from build123d import *

# Parameters (mm, degrees)
ESQUISSE1_W             = 15.74
ESQUISSE1_H             = 2.54
BOSS_EXTRU_1_DEPTH      = 8.5
ESQUISSE3_W             = 0.626711562
ESQUISSE3_H             = 0.626711562
ENL_V_MAT_EXTRU_3_DEPTH = 8
CHANFREIN3_SIZE         = 0.6
CHANFREIN3_SIZE2        = 0.267137211
ESQUISSE6_W             = 0.75
ESQUISSE6_H             = 0.4
BOSS_EXTRU_3_DEPTH      = 3.2
CONG_1_R                = 0.3


with BuildPart() as part:
    # Esquisse1 → Boss.-Extru.1 (new body)
    with BuildSketch(Plane(origin=(0, 0, 0), x_dir=(1, 0, 0), z_dir=(0, 1, 0))):
        Rectangle(ESQUISSE1_W, ESQUISSE1_H)
    extrude(amount=BOSS_EXTRU_1_DEPTH)

    # Esquisse3 → Enlèv. mat.-Extru.3 (cut)
    with BuildSketch(Plane(origin=(0, 8.5, 0), x_dir=(1, 0, 0), z_dir=(0, 1, 0))):
        with Locations((-6.35, 0)):
            Rectangle(ESQUISSE3_W, ESQUISSE3_H)
        with Locations((-3.81, 0)):
            Rectangle(ESQUISSE3_W, ESQUISSE3_H)
        with Locations((-1.27, 0)):
            Rectangle(ESQUISSE3_W, ESQUISSE3_H)
        with Locations((1.27, 0)):
            Rectangle(ESQUISSE3_W, ESQUISSE3_H)
        with Locations((3.81, 0)):
            Rectangle(ESQUISSE3_W, ESQUISSE3_H)
        with Locations((6.35, 0)):
            Rectangle(ESQUISSE3_W, ESQUISSE3_H)
    extrude(amount=-ENL_V_MAT_EXTRU_3_DEPTH, mode=Mode.SUBTRACT)

    # Chanfrein3
    chanfrein3_edges = [part.edges().sort_by_distance(p)[0] for p in [
        (-3.81, 8.5, -0.313355781),
        (-3.496644219, 8.5, 0),
        (-4.123355781, 8.5, 0),
        (-3.81, 8.5, 0.313355781),
        (-6.35, 8.5, -0.313355781),
        (-6.036644219, 8.5, 0),
        (-6.663355781, 8.5, 0),
        (-6.35, 8.5, 0.313355781),
        (3.81, 8.5, -0.313355781),
        (4.123355781, 8.5, 0),
        (3.496644219, 8.5, 0),
        (3.81, 8.5, 0.313355781),
        (1.27, 8.5, -0.313355781),
        (1.583355781, 8.5, 0),
        (0.956644219, 8.5, 0),
        (1.27, 8.5, 0.313355781),
        (-1.27, 8.5, -0.313355781),
        (-0.956644219, 8.5, 0),
        (-1.583355781, 8.5, 0),
        (-1.27, 8.5, 0.313355781),
        (6.35, 8.5, -0.313355781),
        (6.663355781, 8.5, 0),
        (6.036644219, 8.5, 0),
        (6.35, 8.5, 0.313355781),
    ]]
    chanfrein3_side = [part.faces().sort_by_distance(p)[0] for p in [
        (0, 8.5, 0),
    ]]
    chamfer(chanfrein3_edges, length=CHANFREIN3_SIZE, length2=CHANFREIN3_SIZE2, reference=chanfrein3_side[0])

    # Esquisse6 → Boss.-Extru.3 (add)
    with BuildSketch(Plane.XZ):
        with Locations((-6.35, 0)):
            Rectangle(ESQUISSE6_W, ESQUISSE6_H)
        with Locations((-3.81, 0)):
            Rectangle(ESQUISSE6_W, ESQUISSE6_H)
        with Locations((-1.27, 0)):
            Rectangle(ESQUISSE6_W, ESQUISSE6_H)
        with Locations((1.27, 0)):
            Rectangle(ESQUISSE6_W, ESQUISSE6_H)
        with Locations((3.81, 0)):
            Rectangle(ESQUISSE6_W, ESQUISSE6_H)
        with Locations((6.35, 0)):
            Rectangle(ESQUISSE6_W, ESQUISSE6_H)
    extrude(amount=BOSS_EXTRU_3_DEPTH)

    # Congé1
    cong_1_edges = [part.edges().sort_by_distance(p)[0] for p in [
        (-5.975, -3.2, 0),
        (-6.725, -3.2, 0),
        (-3.435, -3.2, 0),
        (-4.185, -3.2, 0),
        (-0.895, -3.2, 0),
        (-1.645, -3.2, 0),
        (1.645, -3.2, 0),
        (0.895, -3.2, 0),
        (4.185, -3.2, 0),
        (3.435, -3.2, 0),
        (6.725, -3.2, 0),
        (5.975, -3.2, 0),
    ]]
    fillet(cong_1_edges, radius=CONG_1_R)


solid = part.part
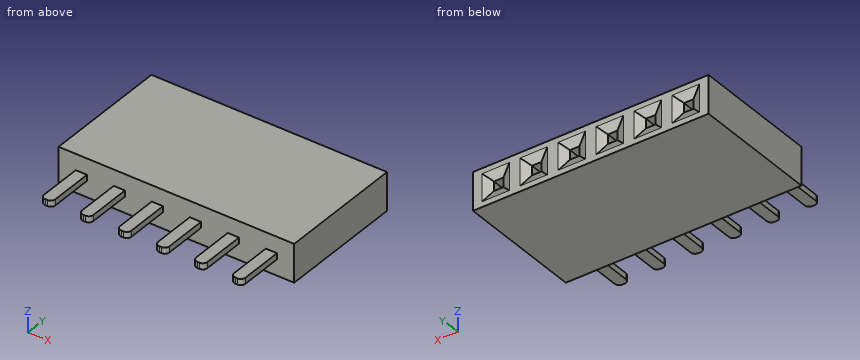
Verification items for the finished model (mm, model axes). Coordinates: 2 decimals unless noted, no trailing zeros. Order: outer loops, then holes, each group sorted by start corner. A loop starts at its lowest first (then second) coordinate and runs counter-clockwise, first axis right, second up. Notation, with made-up numbers: M 13,65.25 L 59,65.25 A31 ccw 59,91.25 Z; hole C 31.25,67 d11. An arc over 180 degrees is marked long. One line per item, written item: value. Start each with the question number.
Item 1: Scan lines: probe 1 along Z at (x, y) = (1.5, 6); probe 2 along Y at (x, z) = (5.75, -1.2); probe 3 along Y at (x, z) = (1.25, 0). Record each from-to range of solid material in increasing order.
Item 2: Sectioned sample at B-B (y = -1.5). Enter the section's corners in (x, z) (3 decimals).
Item 3: Gauge pin test, flat ends, axial feed: pin 1 (0.8 mm diameter, centred on x = 1, y = -1.5, fed in from -Z); pin 2 (0.6 mm diameter, centred on x = 6.5, y = -2, fed in from +Z). Record the tip position at first contact, or that the pin passes through.
Item 4: Sectioned sample at C-C (z = 0.65). Enter the section's corners in (x, y), then the cut area to 3 significant figures.
Item 5: Sectioned sample at A-A (y = 2). Enter the section's corners in (x, z), then the cut area to 3 significant figures.
Conclusion:
1. probe 1: z = -1.27 to -0.31, 0.31 to 1.27
1. probe 2: y = 0 to 8.5
1. probe 3: y = -3.2 to 0.5
2. outline: M -6.725,-0.2 L -5.975,-0.2 L -5.975,0.2 L -6.725,0.2 Z; M -4.185,-0.2 L -3.435,-0.2 L -3.435,0.2 L -4.185,0.2 Z; M -1.645,-0.2 L -0.895,-0.2 L -0.895,0.2 L -1.645,0.2 Z; M 0.895,-0.2 L 1.645,-0.2 L 1.645,0.2 L 0.895,0.2 Z; M 3.435,-0.2 L 4.185,-0.2 L 4.185,0.2 L 3.435,0.2 Z; M 5.975,-0.2 L 6.725,-0.2 L 6.725,0.2 L 5.975,0.2 Z
3. pin 1: stops at z = -0.2
3. pin 2: stops at z = 0.2
4. outline: M -7.87,0 L 7.87,0 L 7.87,8.5 L 7.26,8.5 L 7,8.38 L 5.7,8.38 L 5.44,8.5 L 4.72,8.5 L 4.46,8.38 L 3.16,8.38 L 2.9,8.5 L 2.18,8.5 L 1.92,8.38 L 0.62,8.38 L 0.36,8.5 L -0.36,8.5 L -0.62,8.38 L -1.92,8.38 L -2.18,8.5 L -2.9,8.5 L -3.16,8.38 L -4.46,8.38 L -4.72,8.5 L -5.44,8.5 L -5.7,8.38 L -7,8.38 L -7.26,8.5 L -7.87,8.5 Z
4. area: 133 mm^2
5. outline: M -7.87,-1.27 L 7.87,-1.27 L 7.87,1.27 L -7.87,1.27 Z; hole M -6.66,-0.31 L -6.04,-0.31 L -6.04,0.31 L -6.66,0.31 Z; hole M -4.12,-0.31 L -3.5,-0.31 L -3.5,0.31 L -4.12,0.31 Z; hole M -1.58,-0.31 L -0.96,-0.31 L -0.96,0.31 L -1.58,0.31 Z; hole M 0.96,-0.31 L 1.58,-0.31 L 1.58,0.31 L 0.96,0.31 Z; hole M 3.5,-0.31 L 4.12,-0.31 L 4.12,0.31 L 3.5,0.31 Z; hole M 6.04,-0.31 L 6.66,-0.31 L 6.66,0.31 L 6.04,0.31 Z
5. area: 37.6 mm^2
